Read the model definition and answer for the solid it produces. Units are mm, in the model's axes. Face numbers are marked on the shaded views. Give positions to 0.01 mm unless a question says otherwise; leave off trailing zeros. Order: outer loops, then holes, each group sorted by start corner. A loop starts at its lowest first (then second) coordinate and runs counter-clockwise, first axis right, second up. Notation, with made-up numbers: M 24,67.25 L 34,67.25 A29 cw 34,94.25 Z; hole C 28,19.5 d3. An arc over 180 degrees is marked long. One line per item, written item: value.
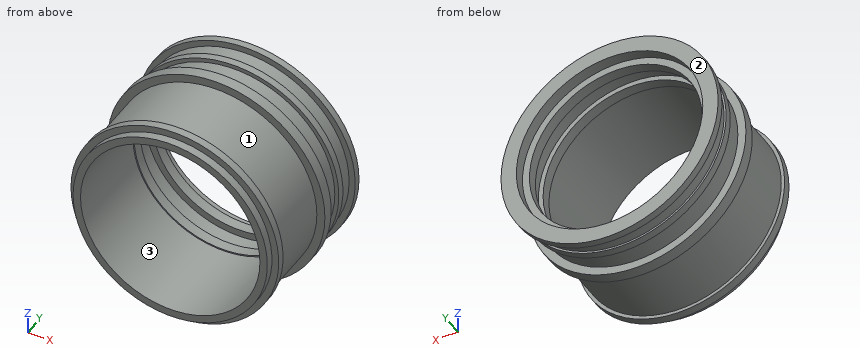
from build123d import *


with BuildPart() as part:
    # Sketch1 → Revolve1 (revolve)
    with BuildSketch(Plane.XY):
        Polygon((-75.784806401, 0), (-75.784806401, 6.356320182), (-81.037271199, 6.356320182), (-81.037271199, 12.359137093), (-78.4110388, 12.359137093), (-78.4110388, 63.243015116), (-84.710995149, 63.243015116), (-84.710995149, 71.887071469), (-78.4110388, 71.887071469), (-78.4110388, 87.878575722), (-81.561016974, 87.878575722), (-81.561016974, 93.497212352), (-79.986027887, 93.497212352), (-79.986027887, 104.734485611), (-84.710995149, 104.734485611), (-84.710995149, 110), (-72.728358467, 110), (-72.728358467, 101.639947534), (-67.271641533, 101.639947534), (-67.271641533, 93.497212352), (-72.728358467, 93.497212352), (-72.728358467, 79.882823596), (-69, 79.882823596), (-69, 71.887071469), (-70, 71.887071469), (-70, 0), align=None)
    revolve(axis=Axis((0, -0.310935058, 0), (0, 1, 0)))


solid = part.part
1) Consider probe 1 along Z at (x, y) = (0, 74.5); probe 2 along Z at (x, y) = (0, 107); probe 3 along X at (y, z) = (90.5, -28.5). Determine where each line is inside the solid, lowest interval first.
Reported:
probe 1: z = -78.41 to -69, 69 to 78.41
probe 2: z = -84.71 to -72.73, 72.73 to 84.71
probe 3: x = -76.42 to -66.91, 66.91 to 76.42
2) Each of these flat-tipped pins is pushed along its axis until it touches: pin 1 Ø2 at (x, y) = (-24.5, 11.5) entering from +Z; pin 2 Ø5 at (x, z) = (-31, -60.5) entering from -Y; pin 3 Ø1.5 at (y, z) = (81, -8.5) entering from +X; pin 4 Ø3 at (y, z) = (48, -60) entering from -X. Where does it stop, or does it pass through?
Reported:
pin 1: stops at z = 77.56
pin 2: stops at y = 0
pin 3: stops at x = 78.03
pin 4: stops at x = -52.21
3) Find section A-A, the plane y = 31.5. Write down the section's boundary in (x, z).
Reported:
outline: C 0,0 d156.82; hole C 0,0 d140
4) Determine the mould class of the marked faces 1, 2 and 3 for opening direction Z: +Z half, -Z half, draft (parallel to the pull), parting line (faces both ways), or undercut.
Reported:
face 1: parting line
face 2: draft
face 3: undercut
